from build123d import *

# Parameters (mm, degrees)
SKETCH1_R           = 12.7
BOSS_EXTRUDE1_DEPTH = 2.38125
CUT_EXTRUDE1_DEPTH  = 5.7625
FILLET1_R           = 3.175
SKETCH3_RX          = 21.59
SKETCH3_RY          = 20.32
CUT_EXTRUDE2_DEPTH  = 5.7625
CIRPATTERN1_COUNT   = 6
SKETCH4_R           = 1.27
CUT_EXTRUDE3_DEPTH  = 5.7625001
CIRPATTERN2_COUNT   = 6


with BuildPart() as part:
    # Sketch1 → Boss-Extrude1 (new body, symmetric)
    with BuildSketch(Plane(origin=(0, 0, 0), x_dir=(1, 0, 0), z_dir=(0, 1, 0))):
        with BuildLine():
            Line((-60.1472, 5.553404471), (-60.1472, 9.525))
            Line((-60.1472, 9.525), (-38.322491971, 47.326503167))
            Line((-38.322491971, 47.326503167), (-34.88298935, 49.312300931))
            ThreePointArc((-34.88298935, 49.312300931), (-27.384375, 47.431128834), (-25.26421065, 54.865705402))
            Line((-25.26421065, 54.865705402), (-21.824708029, 56.851503167))
            Line((-21.824708029, 56.851503167), (21.824708029, 56.851503167))
            Line((21.824708029, 56.851503167), (25.26421065, 54.865705402))
            ThreePointArc((25.26421065, 54.865705402), (27.384375, 47.431128834), (34.88298935, 49.312300931))
            Line((34.88298935, 49.312300931), (38.322491971, 47.326503167))
            Line((38.322491971, 47.326503167), (60.1472, 9.525))
            Line((60.1472, 9.525), (60.1472, 5.553404471))
            ThreePointArc((60.1472, 5.553404471), (54.76875, 0), (60.1472, -5.553404471))
            Line((60.1472, -5.553404471), (60.1472, -9.525))
            Line((60.1472, -9.525), (38.322491971, -47.326503167))
            Line((38.322491971, -47.326503167), (34.88298935, -49.312300931))
            ThreePointArc((34.88298935, -49.312300931), (27.384375, -47.431128834), (25.26421065, -54.865705402))
            Line((25.26421065, -54.865705402), (21.824708029, -56.851503167))
            Line((21.824708029, -56.851503167), (-21.824708029, -56.851503167))
            Line((-21.824708029, -56.851503167), (-25.26421065, -54.865705402))
            ThreePointArc((-25.26421065, -54.865705402), (-27.384375, -47.431128834), (-34.88298935, -49.312300931))
            Line((-34.88298935, -49.312300931), (-38.322491971, -47.326503167))
            Line((-38.322491971, -47.326503167), (-60.1472, -9.525))
            Line((-60.1472, -9.525), (-60.1472, -5.553404471))
            ThreePointArc((-60.1472, -5.553404471), (-54.76875, 0), (-60.1472, 5.553404471))
        make_face()
        Circle(SKETCH1_R, mode=Mode.SUBTRACT)
    extrude(amount=BOSS_EXTRUDE1_DEPTH, both=True)

    # Sketch2 → Cut-Extrude1 (cut, through all)
    with BuildSketch(Plane(origin=(0, 2.38125, 0), x_dir=(1, 0, 0), z_dir=(0, 1, 0))):
        Polygon((10.61724051, -18.3896), (21.234481021, 0), (10.61724051, 18.3896), (-10.61724051, 18.3896), (-21.234481021, 0), (-10.61724051, -18.3896), align=None)
    extrude(amount=-CUT_EXTRUDE1_DEPTH, mode=Mode.SUBTRACT)

    # Fillet1
    fillet1_edges = [part.edges().sort_by_distance(p)[0] for p in [
        (10.61724051, 0, 18.3896),
        (-10.61724051, 0, 18.3896),
        (-21.234481021, 0, 0),
        (-10.61724051, 0, -18.3896),
        (10.61724051, 0, -18.3896),
        (21.234481021, 0, 0),
    ]]
    fillet(fillet1_edges, radius=FILLET1_R)

    # Sketch3 → Cut-Extrude2 (cut, through all)
    with BuildSketch(Plane(origin=(0, 2.38125, 0), x_dir=(1, 0, 0), z_dir=(0, 1, 0))):
        with Locations(Location((0, -56.851503167), (0, 0, -90))):
            Ellipse(SKETCH3_RX, SKETCH3_RY)
    cut_extrude2 = extrude(amount=-CUT_EXTRUDE2_DEPTH, mode=Mode.SUBTRACT)

    # CirPattern1: Cut-Extrude2 ×6 about axis
    cirpattern1_axis = Axis((0, -2.619375, 0), (0, 1, 0))
    for i in range(1, CIRPATTERN1_COUNT):
        add(cut_extrude2.rotate(cirpattern1_axis, i * 360 / CIRPATTERN1_COUNT), mode=Mode.SUBTRACT)

    # Sketch4 → Cut-Extrude3 (cut, through all)
    with BuildSketch(Plane(origin=(0, 2.38125, 0), x_dir=(1, 0, 0), z_dir=(0, 1, 0))):
        with Locations((41.91, 0)):
            Circle(SKETCH4_R)
    cut_extrude3 = extrude(amount=-CUT_EXTRUDE3_DEPTH, mode=Mode.SUBTRACT)

    # CirPattern2: Cut-Extrude3 ×6 about axis
    cirpattern2_axis = Axis((0, 0, 0), (0, 1, 0))
    for i in range(1, CIRPATTERN2_COUNT):
        add(cut_extrude3.rotate(cirpattern2_axis, i * 360 / CIRPATTERN2_COUNT), mode=Mode.SUBTRACT)


solid = part.part
Design review of the part built by this model. Coordinates are the model's own, in mm. A direction names the side the tool comes from. Round coordinates to 2 decimals unless told otherwise and drop trailing zeros. Use a Markdown table: item, result. Add a question column.
1. Wall thickness on probe 1 along X at (y, z) = (0, 0); probe 2 along Z at (x, y) = (-38.5, -2); probe 3 along Z at (x, y) = (49, 1.9): over which ranges is each line inside the solid? List them lowest first.
2. Clearance check with flat-ended pins moving along their axes: pin 1 (1.5 mm diameter, centred on x = -20.96, z = 36.3, fed in from -Y); pin 2 (2 mm diameter, centred on y = 2, z = 41.5, fed in from +X); pin 3 (1 mm diameter, centred on y = -0.5, z = 19.5, fed in from -X); pin 4 (1.5 mm diameter, centred on y = 1, z = 39.5, fed in from +X). State where each tip first meets the part, or that it passes through.
3. We need section A-A (y = -1.25). Count the separate pieces of the cut face and the enclosed holes in it, then the cut area to 3 significant figures.
4. Mouldability with a two-part tool opening along Z and no side actions: class faces 3 (the face through (-36.627, 0.033, -48.306)), 4 (the face through (15.864, 0.033, 9.301)), 5 (the face through (-54.77, 0.03, 0.12)), 6 (the face through (36.627, 0.033, 48.306)) as +Z half, -Z half, draft (parallel to the pull), parting line (faces both ways), or undercut.
5. For faces 1 (the face through (-15.987, 0.033, 9.088)), 2 (the face through (-36.579, 0.033, 48.333)), list the 3-axis set-ups (+Z, -Z, +X, -X, +Y, -Y) from which the entire face can be reached by the end or side of a thin tool; tool diameter is ignored.
Output:
| question | item | result |
|---|---|---|
| 1 | probe 1 | x = -54.77 to -43.18, -40.64 to -20.74, 20.74 to 40.64, 43.18 to 54.77 |
| 1 | probe 2 | z = -47.02 to -45.68, -10.08 to 10.08, 45.68 to 47.02 |
| 1 | probe 3 | z = -7.8 to 7.8 |
| 2 | pin 1 | passes through |
| 2 | pin 2 | stops at x = 34.45 |
| 2 | pin 3 | stops at x = -29.82 |
| 2 | pin 4 | stops at x = 32.45 |
| 3 | separate pieces | 1 |
| 3 | enclosed holes | 7 |
| 3 | area | 5,270 mm2 |
| 4 | face 3 | -Z half |
| 4 | face 4 | undercut |
| 4 | face 5 | undercut |
| 4 | face 6 | +Z half |
| 5 | face 1 | +Y, -Y |
| 5 | face 2 | +Z, -X, +Y, -Y |
